CAD build for the part. Positions are in the model's coordinates, mm. A direction names the side the tool comes from. Round coordinates to 2 decimals unless told otherwise and drop trailing zeros. Loops run counter-clockwise (first coordinate to the right, second up) from the corner with the lowest first, then second, coordinate; pieces in that order, holes last. Notation, with made-up numbers: (88, 5.5) - (115, 5.5) arc R22 cw to (115, 29.5) - close; hole circle Ø7 at (-27, 89.25). An arc over 180 degrees is marked (long way). Use one line per item in the form item = value.
Autodesk Inventor part; units mm, degrees
ref_plane "YZ Plane" through (0, 0, 0) normal (1, 0, 0) x (0, 1, 0)
ref_plane "XZ Plane" through (0, 0, 0) normal (0, 1, 0) x (-1, 0, 0)
ref_plane "XY Plane" through (0, 0, 0) normal (0, 0, 1) x (1, 0, 0)
sketch "Sketch1" plane through (0, 0, 0) normal (0, 0, 1) x (1, 0, 0)
  line L0 (0, 0) -> (190, 0)
  line L1 (190, 0) -> (190, 400)
  line L2 (190, 400) -> (0, 400)
  line L3 (0, 400) -> (0, 0)
  dimension "d0" = 190
  dimension "d1" = 400
extrude "Extrusion1" add sketch "Sketch1" along normal blind 20
sketch "Sketch2" plane through (0, 0, 20) normal (0, 0, 1) x (1, 0, 0)
  circle A0 centre (95, 328.575) radius 5 construction
  circle A1 centre (95, 309.525) radius 5 construction
  arc A2 (110, 328.575) -> (80, 328.575) centre (95, 328.575) ccw construction
  arc A3 (80, 309.525) -> (110, 309.525) centre (95, 309.525) ccw construction
  line L0 (95, 309.525) -> (110, 309.525) construction
  line L1 (95, 309.525) -> (80, 309.525) construction
  line L2 (80, 309.525) -> (80, 328.575)
  line L3 (110, 328.575) -> (110, 309.525)
  arc A4 (110, 328.575) -> (80, 328.575) centre (95, 328.575) ccw
  arc A5 (80, 309.525) -> (110, 309.525) centre (95, 309.525) ccw
  point P0 (0, 0)
  dimension "d4" = 15
  dimension "d5" = 15
  dimension "d6" = 180
extrude "Extrusion2" cut sketch "Sketch2" against normal blind 20
equation "\"d0\" = maxw - 4 * nutdist"
equation "\"d1\" = maxh"
equation "\"d2\" = supt"
equation "\"d7\" = supt"
equation "\"maxh\" = 400"
equation "\"lcsd\" = 19.05"
equation "\"lcwd1\" = 25"
equation "\"lcwd2\" = 34"
equation "\"lch1\" = 39"
equation "\"lcwd3\" = 43"
equation "\"dia1\" = 6"
equation "\"td\" = 18"
equation "\"bhh\" = 6"
equation "\"sw\" = 25"
equation "\"sh\" = 31"
equation "\"spacert\" = 2"
equation "\"supt\" = 20"
equation "\"pvct\" = 5"
equation "\"dia3\" = 8"
equation "\"dia4\" = 11"
equation "\"tankl\" = 379"
equation "\"play\" = 9"
equation "\"holeh\" = 26"
equation "\"surroundt\" = 5"
equation "\"slack\" = 0.5"
equation "\"play2\" = 3"
equation "\"diacucl\" = 32"
equation "\"diaoverflow\" = 25"
equation "\"diawater\" = 25"
equation "\"diaph\" = 32"
equation "\"diaair\" = 32"
equation "\"diasurroundhole\" = 42"
equation "\"diagrate\" = 12"
equation "\"gratespacing\" = 12.02082"
equation "\"sidedist\" = 13.9375"
equation "\"bottomdist\" = 9.6355"
equation "\"diahcl\" = 32"
equation "\"bracketwtop\" = 6"
equation "\"bracketwbottom\" = 6"
equation "\"nett\" = 1"
equation "\"nethole\" = 16"
equation "\"nettop\" = 7"
equation "\"netside\" = 3.5"
equation "\"netholespacing\" = 2"
equation "\"diaetape\" = 32"
properties part number "support plate" material "PVC-Piping"
1) Slice it at B-B (z = 6.75). Write the cut outline in (x, y) (3 decimals).
Report:
outline = (0, 0) - (190, 0) - (190, 400) - (0, 400) - close; hole (80, 309.525) arc R15 ccw to (110, 309.525) - (110, 328.575) arc R15 ccw to (80, 328.575) - close
2) Slice it at C-C (y = 314). Write the cut outline in (x, z).
Report:
outline = (0, 0) - (80, 0) - (80, 20) - (0, 20) - close; (110, 0) - (190, 0) - (190, 20) - (110, 20) - close
3) Slice it at A-A (x = 95). Write the cut outline in (y, z) (3 decimals), plus the area to 3 significant figures.
Report:
outline = (0, 0) - (294.525, 0) - (294.525, 20) - (0, 20) - close; (343.575, 0) - (400, 0) - (400, 20) - (343.575, 20) - close
area = 7,020 mm^2
4) Tool access for faces 5 (the flat face through (110, 319, 10)), 6 (the flat face through (94, 203, 0)): list every direction of +Z, -Z, +X, -X, +Y, -Y with a clear straight run to the whole face (end or side of a thin tool).
Report:
face_5 = +Z, -Z
face_6 = -Z, +X, -X, +Y, -Y
5) Drill centre lines: probe 1 along X at (y, z) = (307, 3.25); probe 2 along Y at (x, z) = (82, 11.75); probe 3 along Y at (x, z) = (104.5, 7). Where is each one in solid material? Low to high.
Report:
probe_1 = 0 to 80.21, 109.79 to 190
probe_2 = 0 to 302.04, 336.06 to 400
probe_3 = 0 to 297.92, 340.18 to 400
6) Two-plate mould, pull along X, no slides. Class faces 1 (the flat face through (190, 197, 10)), 2 (the flat face through (80, 319, 10)), 3 (the cylindrical face through (95.33, 343.57, 10.14)), 4 (the flat face through (0, 203, 10)): +X half, -X half, draft (parallel to the pull), parting line (faces both ways), or undercut.
Report:
face_1 = +X half
face_2 = undercut
face_3 = undercut
face_4 = -X half
